```python
from build123d import *

# Parameters (mm, degrees)
CYLINDER001_R           = 3.175
CYLINDER001_DEPTH       = 25.4
CYLINDER001_PITCH_ANGLE = 90
CYLINDER_R              = 22.225
CYLINDER_DEPTH          = 50.8
SKETCH_R                = 7.9375
POCKET_DEPTH            = 50.801
SKETCH001_R             = 12.7
POCKET001_DEPTH         = 25.4
SKETCH002_W             = 6.35
SKETCH002_H             = 6.35
PAD_DEPTH               = 25.4


with BuildPart() as cylinder001:
    # Cylinder001 → Cylinder001 (new body)
    with BuildSketch(Plane.XY):
        Circle(CYLINDER001_R)
    extrude(amount=CYLINDER001_DEPTH)


with BuildPart() as cylinder001_1:
    # Cylinder001 pitch: moved
    add(cylinder001.part.rotate(Axis((0, 0, 0), (0, 1, 0)), CYLINDER001_PITCH_ANGLE))


with BuildPart() as cylinder001_2:
    # Cylinder001 placement: moved
    add(cylinder001_1.part.moved(Location((1.93153, 0, 12.7))))


with BuildPart() as f_0_25in_key:
    # Cylinder → Cylinder (new body)
    with BuildSketch(Plane.XY):
        Circle(CYLINDER_R)
    extrude(amount=CYLINDER_DEPTH)

    # Sketch → Pocket (cut, through all)
    with BuildSketch(Plane.XY.offset(50.8)):
        Circle(SKETCH_R)
    extrude(amount=-POCKET_DEPTH, mode=Mode.SUBTRACT)

    # Cut: cut Cylinder001
    add(cylinder001_2.part, mode=Mode.SUBTRACT)

    # Sketch001 → Pocket001 (cut)
    with BuildSketch(Plane(origin=(0, 0, 0), x_dir=(1, 0, 0), z_dir=(0, 0, -1))):
        Circle(SKETCH001_R)
    extrude(amount=-POCKET001_DEPTH, mode=Mode.SUBTRACT)

    # Sketch002 → Pad (new body)
    with BuildSketch(Plane(origin=(0, 0, 0), x_dir=(1, 0, 0), z_dir=(0, 0, -1))):
        with Locations((12.7, 0)):
            Rectangle(SKETCH002_W, SKETCH002_H)
    extrude(amount=-PAD_DEPTH)


solid = f_0_25in_key.part
```
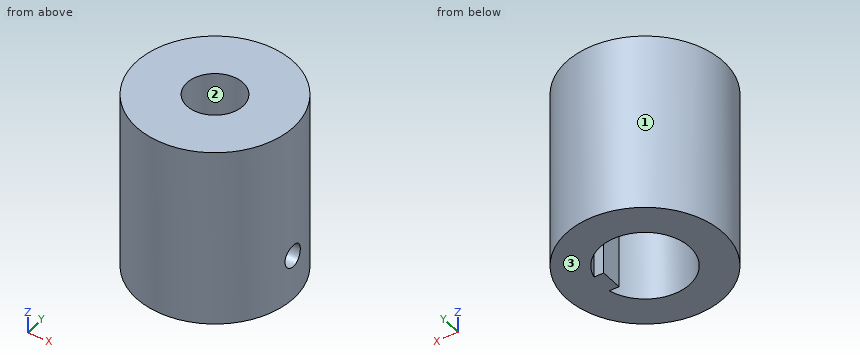
Here's how the part is built. I have some questions about the finished solid (model axes, mm). Face numbers are marked on the shaded views. Give positions to 0.01 mm unless a question says otherwise; leave off trailing zeros. Write each loop counter-clockwise with the first axis right and the second up, starting at its lowest first coordinate (ties: lowest second). Pieces come first, ordered by that corner, then holes. Notation, with made-up numbers: M 48,-10 L 74,-10 A10 ccw 74,1 Z; hole C 87.25,-10 d11. An arc over 180 degrees is marked long. Put each result on its own line as item: value. Start each with the question number.
Item 1: Thinking about a two-plate mould opening in Y: for the marked faces 1, 2 and 3, which applies, +Y half, -Y half, draft (parallel to the pull), parting line (faces both ways), or undercut?
Item 2: If we section it at A-A, the plane y = 0: Write out the boundary of the cut face in (x, z) (1 decimal).
Item 3: If we section it at C-C, the plane z = 13: Write out the boundary of the cut face in (x, y) (3 decimals).
Item 4: Will these pins go through, and if not, where does the flat tip stop? pin 1 (12 mm diameter, centred on y = -8, z = 14.5, fed in from -X); pin 2 (1.5 mm diameter, centred on x = 3, y = 8.5, fed in from -Z); pin 3 (2 mm diameter, centred on y = 2, z = 27.5, fed in from -X).
Item 5: If we section it at D-D, the plane y = -12: Write out the boundary of the cut face in (x, z).
Item 6: I need wall thicknesses on L1, parallel to Y at x = 0, z = 44 (1 decimal); L2, parallel to X at y = -0.5, z = 43; L3, parallel to Z at x = 18.25, y = 0 (3 decimals). Which ranges of each line are inside material? Lowest first, please. Write a range as from..to.
Item 7: If we section it at B-B, the plane x = 0: Write out the boundary of the cut face in (y, z) (1 decimal).
Values:
1. face 1: parting line
1. face 2: undercut
1. face 3: draft
2. outline: M -22.2,0 L -12.7,0 L -12.7,25.4 L -7.9,25.4 L -7.9,50.8 L -22.2,50.8 Z; M 7.9,25.4 L 9.5,25.4 L 9.5,0 L 22.2,0 L 22.2,9.5 L 15.9,9.5 L 15.9,15.9 L 22.2,15.9 L 22.2,50.8 L 7.9,50.8 Z
3. outline: M 15.875,-3.161 L 15.875,3.161 L 21.999,3.161 A22.225 ccw long 21.999,-3.161 Z; hole M 9.525,-3.175 L 9.525,3.175 L 12.297,3.175 A12.7 ccw long 12.297,-3.175 Z
4. pin 1: x = -22.13
4. pin 2: z = 25.4
4. pin 3: x = -22.2
5. outline: M -18.71,0 L -4.16,0 L -4.16,25.4 L 4.16,25.4 L 4.16,0 L 18.71,0 L 18.71,50.8 L -18.71,50.8 Z
6. L1: -22.2..-7.9, 7.9..22.2
6. L2: -22.22..-7.92, 7.92..22.22
6. L3: 0..9.525, 15.875..50.8
7. outline: M -22.2,0 L -12.7,0 L -12.7,25.4 L -7.9,25.4 L -7.9,50.8 L -22.2,50.8 Z; M 7.9,25.4 L 12.7,25.4 L 12.7,0 L 22.2,0 L 22.2,50.8 L 7.9,50.8 Z
